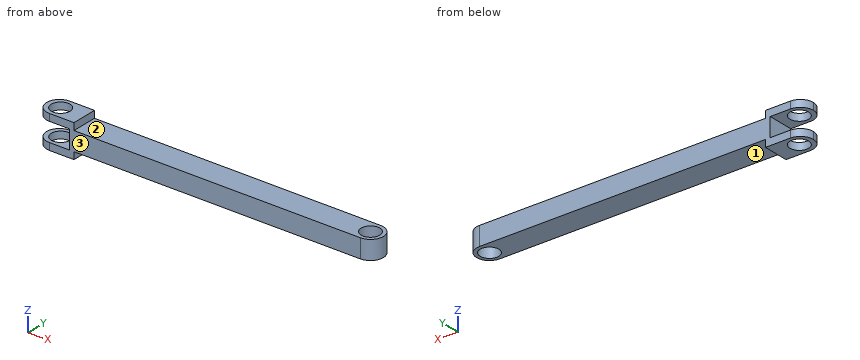
```python
from build123d import *

# Parameters (mm, degrees)
SKETCH1_R               = 2
BOSS_EXTRUDE1_DEPTH     = 4
SKETCH2_W               = 7
SKETCH2_H               = 5.5
BOSS_EXTRUDE2_DEPTH     = 8
CUT_EXTRUDE1_DEPTH      = 70.024452189
CUT_EXTRUDE1_DEPTH_BACK = 70.024452189
SKETCH4_W               = 7
SKETCH4_H               = 4
CUT_EXTRUDE2_DEPTH      = 70.024452189
CUT_EXTRUDE2_DEPTH_BACK = 70.024452189
SKETCH5_R               = 2
FILLET1_R               = 2.75


with BuildPart() as part:
    # Sketch1 → Boss-Extrude1 (new body)
    with BuildSketch(Plane.XY):
        with BuildLine():
            Line((0, 2.75), (-60.75, 2.75))
            Line((-60.75, 2.75), (-60.75, -2.75))
            Line((-60.75, -2.75), (0, -2.75))
            ThreePointArc((0, -2.75), (2.75, 0), (0, 2.75))
        make_face()
        Circle(SKETCH1_R, mode=Mode.SUBTRACT)
    extrude(amount=BOSS_EXTRUDE1_DEPTH)

    # Sketch2 → Boss-Extrude2 (add)
    with BuildSketch(Plane.ZY.offset(60.75)):
        with Locations((2, 0)):
            Rectangle(SKETCH2_W, SKETCH2_H)
    extrude(amount=BOSS_EXTRUDE2_DEPTH)

    # Sketch4 → Cut-Extrude1 (cut, two sides: drawn at the far end of the back side and taken through both)
    with BuildSketch(Plane(origin=(0, 0, 0), x_dir=(1, 0, 0), z_dir=(0, 1, 0)).offset(-CUT_EXTRUDE1_DEPTH_BACK)):
        with Locations((-65.25, -2)):
            Rectangle(SKETCH4_W, SKETCH4_H)
    extrude(amount=CUT_EXTRUDE1_DEPTH + CUT_EXTRUDE1_DEPTH_BACK, mode=Mode.SUBTRACT)

    # Sketch5 → Cut-Extrude2 (cut, two sides: drawn at the far end of the back side and taken through both)
    with BuildSketch(Plane.XY.offset(-CUT_EXTRUDE2_DEPTH_BACK)):
        with Locations((-65.75, 0)):
            Circle(SKETCH5_R)
    extrude(amount=CUT_EXTRUDE2_DEPTH + CUT_EXTRUDE2_DEPTH_BACK, mode=Mode.SUBTRACT)

    # Fillet1
    fillet1_edges = [part.edges().sort_by_distance(p)[0] for p in [
        (-68.75, -2.75, 4.75),
        (-68.75, -2.75, -0.75),
        (-68.75, 2.75, -0.75),
        (-68.75, 2.75, 4.75),
    ]]
    fillet(fillet1_edges, radius=FILLET1_R - 0.0001)  # a hair under: the kernel refuses the full size


solid = part.part
```
Part model, mm, in its own coordinate system. Face numbers are marked on the shaded views. A direction names the side the tool comes from. Give positions to 0.01 mm unless a question says otherwise; leave off trailing zeros. Order: outer loops, then holes, each group sorted by start corner. A loop starts at its lowest first (then second) coordinate and runs counter-clockwise, first axis right, second up. Notation, with made-up numbers: M 30,60.25 L 46,60.25 A17 cw 46,66.25 Z; hole C 82,-30 d7. An arc over 180 degrees is marked long. Use a Markdown table: item, result. Add a question column.
(1) Drop flat-ended pins along their axis: P1, Ø1, axis at y = 1.5, z = 2.5, coming from the -X side; P2, Ø3, axis at x = -9, y = 0.5, coming from the +Z side; P3, Ø2, axis at y = 0.5, z = 1, coming from the +X side; P4, Ø3, axis at x = -33.5, y = 0, coming from the -Z side. Give the stop position or say it passes through.
(2) Saw through at A-A, the plane x = -63. Give the cut face in (y, z), and give its area (3 significant figures).
(3) 3-axis set-ups, long thin cutter, end or side, ignore diameter. For the marked faces 1, 2 and 3: which of +Z, -Z, +X, -X, +Y, -Y reach the whole face in a straight line?
(4) Saw through at B-B, the plane z = 0.75. Give the cut face in (x, y), and give its area (3 significant figures).
(5) Saw through at C-C, the plane y = 1.15. Give the cut face in (x, z).
(6) Probe line 1 along X through (y, z) = (0, -0.55); line 2 along Y through (x, z) = (-65.75, 5); line 3 along Z through (x, y) = (-63, 1.55). List the from-to ranges inside material, lowest first. Write a range as [from, to].
(7) Saw through at D-D, the plane x = -39. Give the cut face in (y, z).
Answer key:
| question | item | result |
|---|---|---|
| 1 | P1 | x = -61.75 |
| 1 | P2 | z = 4 |
| 1 | P3 | x = 2.75 |
| 1 | P4 | z = 0 |
| 2 | outline | M -2.75,-1.5 L 2.75,-1.5 L 2.75,0 L -2.75,0 Z; M -2.75,4 L 2.75,4 L 2.75,5.5 L -2.75,5.5 Z |
| 2 | area | 16.5 mm^2 |
| 3 | face 1 | -Z, +X, +Y, -Y |
| 3 | face 2 | +Z, +X, +Y, -Y |
| 3 | face 3 | +Z, -Z, +X, -X, -Y |
| 4 | outline | M -61.75,-2.75 L 0,-2.75 A2.75 ccw 0,2.75 L -61.75,2.75 Z; hole C 0,0 d4 |
| 4 | area | 339 mm^2 |
| 5 | outline | M -68.5,-1.5 L -67.39,-1.5 L -67.39,0 L -68.5,0 Z; M -68.5,4 L -67.39,4 L -67.39,5.5 L -68.5,5.5 Z; M -64.11,-1.5 L -60.75,-1.5 L -60.75,0 L -1.64,0 L -1.64,4 L -60.75,4 L -60.75,5.5 L -64.11,5.5 L -64.11,4 L -61.75,4 L -61.75,0 L -64.11,0 Z; M 1.64,0 L 2.5,0 L 2.5,4 L 1.64,4 Z |
| 6 | line 1 | [-68.75, -67.75], [-63.75, -60.75] |
| 6 | line 2 | [-2.75, -2], [2, 2.75] |
| 6 | line 3 | [-1.5, 0], [4, 5.5] |
| 7 | outline | M -2.75,0 L 2.75,0 L 2.75,4 L -2.75,4 Z |
